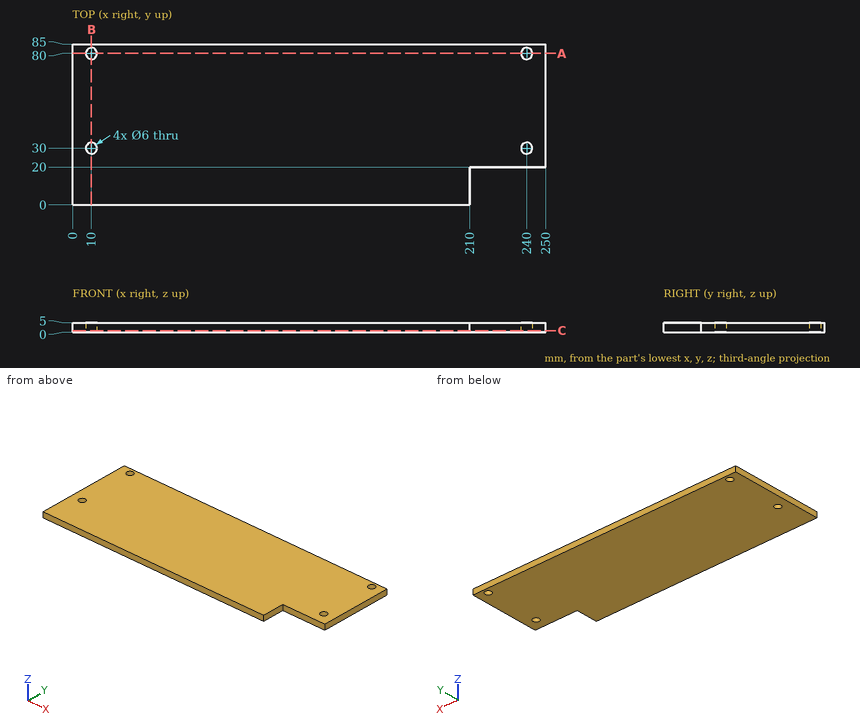
Check sheet for the drawn part. Datum: minimum x, y, z corner. Units: mm. Coordinates: 2 decimals unless noted, no trailing zeros. Order: outer loops, then holes, each group sorted by start corner. A loop starts at its lowest first (then second) coordinate and runs counter-clockwise, first axis right, second up. Notation, with made-up numbers: M -29.75,45 L 14.25,45 A5 ccw 14.25,53 Z; hole C 8.5,-25 d3. An arc over 180 degrees is marked long. One line per question, with ' | ' between items. Start each with the question number.
Item 1: Cross-section at B-B on x = 10. Enter the section's corners in (y, z), then the cut area to 3 significant figures.
Item 2: Cross-section at A-A on y = 80. Enter the section's corners in (x, z), then the cut area to 3 significant figures.
Item 3: Cross-section at C-C on z = 0.9. Enter the section's corners in (x, y).
Item 4: Material ranges on L1, parallel to Y at x = 10, z = 3.9; L2, parallel to Y at x = 240, z = 3.2; L3, parallel to X at y = 79, z = 0.3, recorded low to high. Write a range as [from, to].
Findings:
1) outline: M 0,0 L 27,0 L 27,5 L 0,5 Z; M 33,0 L 77,0 L 77,5 L 33,5 Z; M 83,0 L 85,0 L 85,5 L 83,5 Z | area: 365 mm²
2) outline: M 0,0 L 7,0 L 7,5 L 0,5 Z; M 13,0 L 237,0 L 237,5 L 13,5 Z; M 243,0 L 250,0 L 250,5 L 243,5 Z | area: 1,190 mm²
3) outline: M 0,0 L 210,0 L 210,20 L 250,20 L 250,85 L 0,85 Z; hole C 10,30 d6; hole C 10,80 d6; hole C 240,30 d6; hole C 240,80 d6
4) L1: y = [0, 27], [33, 77], [83, 85] | L2: y = [20, 27], [33, 77], [83, 85] | L3: x = [0, 7.17], [12.83, 237.17], [242.83, 250]
